from build123d import *

# Parameters (mm, degrees)
F2_R           = 0.85
F3_DEPTH       = 10
F2_W           = 3
F2_H           = 5
F4_DEPTH       = 15
F6_R           = 1
F7_D           = 4
F7_CBORE_D     = 7.2
F7_CBORE_DEPTH = 3.9
F8_D           = 4
F8_DEPTH       = 20
F8_CSINK_D     = 8
F8_CSINK_ANGLE = 90
F8_TIP         = 1.2017212381
F5_W           = 5
F5_H           = 3
F9_DEPTH       = 14


# Not quite as in the source:
# - a feature of the source that left no trace in its solid (it failed there, or was rolled back) is left out


with BuildPart() as f1:
    # F0 (on Front) → F1 (revolve)
    with BuildSketch(Plane.XZ):
        Polygon((0, 22.0396561921), (-30, 22.0396561921), (-30, 2.0396561921), (0, 2.0396561921), (0, 4.0396561921), (-1, 4.0396561921), (-1, 5.5396561921), (0, 5.5396561921), (0, 10.0396561921), (-2, 10.0396561921), (-2, 12.0396561921), (0, 12.0396561921), (0, 18.0396561921), (-3, 18.0396561921), (-3, 19.0396561921), (0, 19.0396561921), align=None)
    revolve(axis=Axis((-30, 0, 12.0396561921), (0, 0, -1)))

    # F2 (on face) → F3 (cut)
    with BuildSketch(Plane.XY.offset(22.0396561921)):
        with BuildLine():
            ThreePointArc((-30.85, 0), (-30, -0.85), (-29.15, 0))
            ThreePointArc((-29.15, 0), (-30, 0.85), (-30.85, 0))
        make_face()
        with Locations((-30, 5.7)):
            Circle(F2_R)
        with Locations((-30, 11.4)):
            Circle(F2_R)
        with Locations((-24.3, 0)):
            Circle(F2_R)
        with Locations((-24.3, 5.7)):
            Circle(F2_R)
        with Locations((-24.3, 11.4)):
            Circle(F2_R)
        with Locations((-18.6, 0)):
            Circle(F2_R)
        with Locations((-18.6, 5.7)):
            Circle(F2_R)
        with Locations((-18.6, 11.4)):
            Circle(F2_R)
    extrude(amount=-F3_DEPTH, mode=Mode.SUBTRACT)

    # F2 (on face) → F4 (join)
    with BuildSketch(Plane.XY.offset(22.0396561921)):
        with Locations((-21.5, -12.5)):
            Rectangle(F2_W, F2_H)
        with Locations((-38.5, -12.5)):
            Rectangle(F2_W, F2_H)
    extrude(amount=F4_DEPTH)

    # F6
    f6_edges = [f1.edges().sort_by_distance(p)[0] for p in [
        (-38.5, -10, 37.039656),
        (-40, -12.5, 37.039656),
        (-38.5, -15, 37.039656),
        (-37, -12.5, 37.039656),
        (-23, -12.5, 37.039656),
        (-21.5, -15, 37.039656),
        (-20, -12.5, 37.039656),
        (-21.5, -10, 37.039656),
    ]]
    fillet(f6_edges, radius=F6_R)

    # F7 (through all)
    with Locations(Plane.XY.offset(22.0396561921)):
        with Locations((-45, 0)):
            CounterBoreHole(F7_D / 2, F7_CBORE_D / 2, F7_CBORE_DEPTH)

    # F8
    with Locations(Plane.XY.offset(22.0396561921)):
        with Locations((-45, 10)):
            CounterSinkHole(F8_D / 2, F8_CSINK_D / 2, depth=F8_DEPTH, counter_sink_angle=F8_CSINK_ANGLE)
            with Locations((0, 0, -(F8_DEPTH + F8_TIP / 2))):  # 118° drill point
                Cone(0, F8_D / 2, F8_TIP, mode=Mode.SUBTRACT)

    # F5 (on face) → F9 (join)
    with BuildSketch(Plane.YZ.offset(-37)):
        with Locations((-12.5, 32.5396561921)):
            Rectangle(F5_W, F5_H)
    extrude(amount=F9_DEPTH)


solid = f1.part
Source: CAD feature listing. Evaluate the final solid. Frame: model axes, mm. A direction names the side the tool comes from. Round coordinates to 2 decimals unless told otherwise and drop trailing zeros. Order: outer loops, then holes, each group sorted by start corner. A loop starts at its lowest first (then second) coordinate and runs counter-clockwise, first axis right, second up. Notation, with made-up numbers: (31, 86) -> (77, 86) arc R29 ccw to (77, 119) -> close; hole circle Ø2 at (-24.5, -14). An arc over 180 degrees is marked (long way). Answer as CSV lines item,"result".
Item 1: Reachability of faces 4 (the face through (-54, 18, 15)), 5 (the face through (-23.49, 5.96, 17.11)), 6 (the face through (-20, -13, 29)) from +Z, -Z, +X, -X, +Y, -Y: full face, straight path, thin tool, end or side. Return the list, or none.
A:
face 4,"+Z, -Z"
face 5,"+Z"
face 6,"+Z, +X, +Y, -Y"
Item 2: Pull-direction query (Y, two-part tool) for faces 1 (the face through (-23.49, 11.66, 17.11)), 2 (the face through (-5.06, 10.34, 18.55)), 3 (the face through (-5, -13, 12.04)); classes: pulls with the +Y half, pulls with the -Y half, needs draft (parallel to the pull), parting line crosses it, or undercut.
A:
face 1,"undercut"
face 2,"parting line crosses it"
face 3,"needs draft"
Item 3: Section C-C, the plane x = -51.5. Return loops of the section in (y, z).
A:
outline,"(-20.92, 2.04) -> (20.92, 2.04) -> (20.92, 4.04) -> (19.46, 4.04) -> (19.46, 5.54) -> (20.92, 5.54) -> (20.92, 10.04) -> (17.94, 10.04) -> (17.94, 12.04) -> (20.92, 12.04) -> (20.92, 18.04) -> (16.33, 18.04) -> (16.33, 19.04) -> (20.92, 19.04) -> (20.92, 22.04) -> (-20.92, 22.04) -> (-20.92, 19.04) -> (-16.33, 19.04) -> (-16.33, 18.04) -> (-20.92, 18.04) -> (-20.92, 12.04) -> (-17.94, 12.04) -> (-17.94, 10.04) -> (-20.92, 10.04) -> (-20.92, 5.54) -> (-19.46, 5.54) -> (-19.46, 4.04) -> (-20.92, 4.04) -> close"
Item 4: Line query: L1, parallel to Y at x = -30, z = 17; L2, parallel to Z at x = -49, y = -23; L3, parallel to X at y = 5, z = 15. Output: solid intervals per line, ascending.
A:
L1,"-30 to -0.85, 0.85 to 4.85, 6.55 to 10.55, 12.25 to 30"
L2,"2.04 to 4.04, 5.54 to 10.04, 12.04 to 18.04, 19.04 to 22.04"
L3,"-59.58 to -30.48, -29.52 to -24.78, -23.82 to -19.08, -18.12 to -0.42"
Item 5: Section D-D, the plane x = -44. Count the separate pieces of the cut face and the enclosed holes in it, plus the area to 4 significant figures.
A:
separate pieces,"3"
enclosed holes,"0"
area,"885.5 mm²"
Item 6: Section B-B, the plane y = 18.5. Return loops of the section in (x, z), plus the area to 3 significant figures.
A:
outline,"(-53.62, 2.04) -> (-6.38, 2.04) -> (-6.38, 4.04) -> (-7.67, 4.04) -> (-7.67, 5.54) -> (-6.38, 5.54) -> (-6.38, 10.04) -> (-8.98, 10.04) -> (-8.98, 12.04) -> (-6.38, 12.04) -> (-6.38, 18.04) -> (-10.33, 18.04) -> (-10.33, 19.04) -> (-6.38, 19.04) -> (-6.38, 22.04) -> (-53.62, 22.04) -> (-53.62, 19.04) -> (-49.67, 19.04) -> (-49.67, 18.04) -> (-53.62, 18.04) -> (-53.62, 12.04) -> (-51.02, 12.04) -> (-51.02, 10.04) -> (-53.62, 10.04) -> (-53.62, 5.54) -> (-52.33, 5.54) -> (-52.33, 4.04) -> (-53.62, 4.04) -> close"
area,"923 mm²"
Item 7: Pin query (flat end, axial travel): pin 1 Ø18 at (x, y) = (-36, 3) entering from +Z; pin 2 Ø1.5 at (x, y) = (-24.3, 5.7) entering from +Z; pin 3 Ø1.5 at (y, z) = (5, 12) entering from +X. Return the tip coordinate at first contact, or that it passes through.
A:
pin 1,"z = 22.04"
pin 2,"z = 12.04"
pin 3,"x = -0.3"
